```python
from build123d import *

# Parameters (mm, degrees)
F0_W     = 44.2396106267
F0_H     = 39.6395683834
F1_DEPTH = 35.0012
F0_W_2   = 10.9982
F2_DEPTH = 9.652
F3_SIZE  = 5.0038
F4_R     = 2.3661353078
F5_DEPTH = 12.7
F6_R     = 9.4407644239
F7_DEPTH = 41.91


with BuildPart() as f1:
    # F0 (on Top) → F1 (new body)
    with BuildSketch(Plane.XY):
        with Locations((-6.1320435831, 32.7550717629)):
            Rectangle(F0_W, F0_H)
    extrude(amount=F1_DEPTH)

    # F0 (on Top) → F2 (join)
    with BuildSketch(Plane.XY):
        with Locations((21.4868617302, 32.7550717629)):
            Rectangle(F0_W_2, F0_H)
        with Locations((-33.7509488964, 32.7550717629)):
            Rectangle(F0_W_2, F0_H)
    extrude(amount=F2_DEPTH)

    # F3
    f3_edges = [f1.edges().sort_by_distance(p)[0] for p in [
        (-6.132044, 12.935288, 35.0012),
    ]]
    chamfer(f3_edges, length=F3_SIZE)

    # F4 (on Right) → F5 (join, symmetric)
    with BuildSketch(Plane.YZ):
        with Locations((21.8015406281, 29.3079074472)):
            Circle(F4_R)
    extrude(amount=F5_DEPTH, both=True)

    # F6 (on Top) → F7 (cut, symmetric)
    with BuildSketch(Plane.XY):
        with Locations((-6.9891391322, 27.6436116546)):
            Circle(F6_R)
    extrude(amount=F7_DEPTH, both=True, mode=Mode.SUBTRACT)


solid = f1.part
```
Work out the finished part from the listing and answer in its coordinate system (mm). A direction names the side the tool comes from. Give positions to 0.01 mm unless a question says otherwise; leave off trailing zeros. Write each loop counter-clockwise with the first axis right and the second up, starting at its lowest first coordinate (ties: lowest second). Pieces come first, ordered by that corner, then holes. Notation, with made-up numbers: (51.5, -31.75) -> (79.5, -31.75) arc R19 ccw to (79.5, -15.75) -> close; hole circle Ø5 at (-9.75, -26.75). An arc over 180 degrees is marked (long way). Write item = value, one per line.
Q1. Section D-D on z = 32.5 is taken. Determine the outline of the cut face in (x, y), and give its area (3 significant figures).
Computed values:
outline = (-28.25, 15.44) -> (15.99, 15.44) -> (15.99, 52.57) -> (-28.25, 52.57) -> close; hole circle Ø18.88 at (-6.99, 27.64)
area = 1,360 mm^2
Q2. Flat-ended cylindrical pins translate along their axes: pin 1 Ø4 at (y, z) = (22, 17) entering from +X; pin 2 Ø1.5 at (x, y) = (17, 45.5) entering from +Z; pin 3 Ø12.5 at (y, z) = (24, 16) entering from -X. Find the tip coordinate at first contact, or state that the pin passes through.
Computed values:
pin_1 = 15.99
pin_2 = 9.65
pin_3 = -28.25
Q3. Section A-A on y = 23 is taken. Determine the outline of the cut face in (x, z), and give its area (3 significant figures).
Computed values:
outline = (-39.25, 0) -> (-15.21, 0) -> (-15.21, 35) -> (-28.25, 35) -> (-28.25, 9.65) -> (-39.25, 9.65) -> close; (1.23, 0) -> (26.99, 0) -> (26.99, 9.65) -> (15.99, 9.65) -> (15.99, 35) -> (1.23, 35) -> close
area = 1,190 mm^2
Q4. Section C-C on y = 45 is taken. Determine the outline of the cut face in (x, z), and give its area (3 significant figures).
Computed values:
outline = (-39.25, 0) -> (26.99, 0) -> (26.99, 9.65) -> (15.99, 9.65) -> (15.99, 35) -> (-28.25, 35) -> (-28.25, 9.65) -> (-39.25, 9.65) -> close
area = 1,760 mm^2
Q5. Consider line 1 along X through (y, z) = (25, 22); line 2 along X through (y, z) = (32.5, 20.5); line 3 along X through (y, z) = (42, 26). Determine where each line is inside the solid, lowest interval first.
Computed values:
line_1 = -28.25 to -16.05, 2.07 to 15.99
line_2 = -28.25 to -15.09, 1.11 to 15.99
line_3 = -28.25 to 15.99
Q6. For a pull along Y with two mould halves and no side action, classify faces 1 (the cylindrical face through (-9.04, 18.43, 17.75)), 2 (the flat face through (-7, 52.575, 17)), 3 (the flat face through (-6.44, 15.47, 32.53)), 4 (the flat face through (-34, 33, 9.652)) as pulls with the +Y half, pulls with the -Y half, needs draft (parallel to the pull), parting line crosses it, or undercut.
Computed values:
face_1 = undercut
face_2 = pulls with the +Y half
face_3 = pulls with the -Y half
face_4 = needs draft
Q7. A tool of negligible diameter and unlimited length cuts with its end or side. For faces 5 (the flat face through (21, 33, 9.652)), 6 (the flat face through (-6, 39, 35.001)), 7 (the flat face through (-28.252, 32, 22)), from which of +Z, -Z, +X, -X, +Y, -Y can it reach the whole face along a straight path? Write none if from no direction.
Computed values:
face_5 = +Z, +X, +Y, -Y
face_6 = +Z, +X, -X, +Y, -Y
face_7 = +Z, -X, +Y, -Y
Q8. Section B-B on x = -3 is taken. Determine the outline of the cut face in (y, z).
Computed values:
outline = (12.94, 0) -> (19.09, 0) -> (19.09, 35) -> (17.94, 35) -> (12.94, 30) -> close; (36.2, 0) -> (52.57, 0) -> (52.57, 35) -> (36.2, 35) -> close
